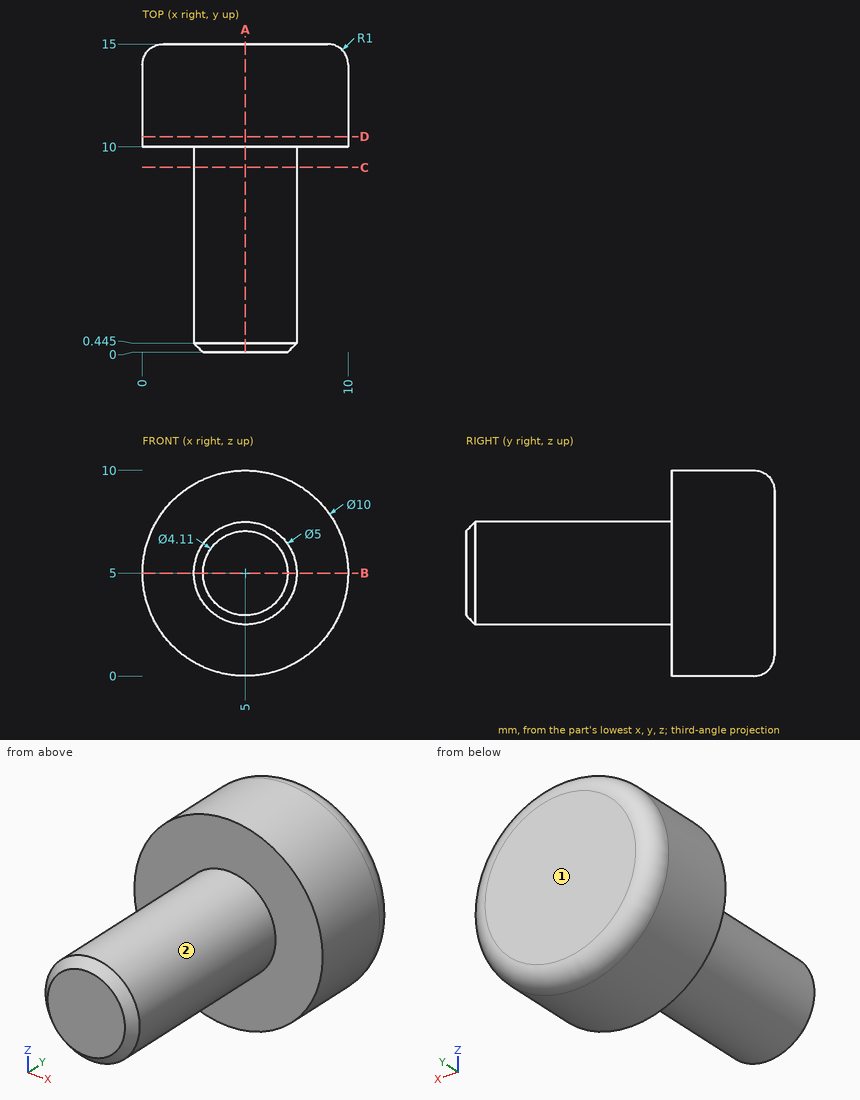
Part print with two shaded views. Sizes in mm from the minimum x, y, z corner. A direction names the side the tool comes from. Round coordinates to 2 decimals unless told otherwise and drop trailing zeros. Order: outer loops, then holes, each group sorted by start corner. A loop starts at its lowest first (then second) coordinate and runs counter-clockwise, first axis right, second up. Notation, with made-up numbers: M 59,-30 L 111,-30 A29 cw 111,-8 Z; hole C 38,39 d5. An arc over 180 degrees is marked long. Use CSV: the item, a comma, the result in double quotes.
Item 1: Saw through at D-D (y = 10.5). List the corners of the cut face in (x, z), plus the area to 3 significant figures.
Worked answers:
outline,"C 5,5 d10"
area,"78.5 mm²"
Item 2: Which spindle directions (+Z, -Z, +X, -X, +Y, -Y) get a long thin tool onto all of the face, cutting with end or side? Do the marked faces 1 and 2. Say none if no direction does.
Worked answers:
face 1,"+Z, -Z, +X, -X, +Y"
face 2,"-Y"
Item 3: Probe probe 1 along Y at (x, z) = (8.25, 7.25); probe 2 along X at (y, z) = (7.25, 4.25); probe 3 along Z at (x, y) = (8, 12). List the from-to ranges inside material, lowest first.
Worked answers:
probe 1,"10 to 15"
probe 2,"2.62 to 7.38"
probe 3,"1 to 9"
Item 4: Saw through at B-B (z = 5). List the corners of the cut face in (x, y) (3 decimals), plus the area to 3 significant figures.
Worked answers:
outline,"M 0,10 L 2.5,10 L 2.5,0.445 L 2.945,0 L 7.055,0 L 7.5,0.445 L 7.5,10 L 10,10 L 10,14 A1 ccw 9,15 L 1,15 A1 ccw 0,14 Z"
area,"99.4 mm²"
Item 5: Pin check, flat tips, straight feed: pin 1 (6 mm diameter, centred on y = 9, z = 8, fed in from +X); pin 2 (5 mm diameter, centred on x = 1, z = 9, fed in from -Y); pin 3 (6 mm diameter, centred on x = 4.5, y = 4, fed in from +Z). Stop position of each tip, or through.
Worked answers:
pin 1,"x = 10"
pin 2,"y = 10"
pin 3,"z = 7.5"
Item 6: Saw through at C-C (y = 9). List the corners of the cut face in (x, z), plus the area to 3 significant figures.
Worked answers:
outline,"C 5,5 d5"
area,"19.6 mm²"
Item 7: Saw through at A-A (x = 5). List the corners of the cut face in (y, z) (3 decimals).
Worked answers:
outline,"M 0,2.945 L 0.445,2.5 L 10,2.5 L 10,0 L 14,0 A1 ccw 15,1 L 15,9 A1 ccw 14,10 L 10,10 L 10,7.5 L 0.445,7.5 L 0,7.055 Z"
